```python
from build123d import *

# Parameters (mm, degrees)
F0_W     = 19.05
F0_H     = 101.6
F1_DEPTH = 9.525
F3_D     = 6.35
F5_D     = 6.35
F7_D     = 6.35


with BuildPart() as f1:
    # F0 (on Right) → F1 (new body, symmetric)
    with BuildSketch(Plane.YZ):
        Rectangle(F0_W, F0_H)
    extrude(amount=F1_DEPTH, both=True)

    # F3 (through all)
    with Locations(Plane.XZ.offset(9.525)):
        with Locations((0, 31.75), (0, -31.75)):
            Hole(F3_D / 2)

    # F5 (through all)
    with Locations(Plane.YZ.offset(9.525)):
        with Locations((0, 41.275), (0, -41.275)):
            Hole(F5_D / 2)

    # F7 (through all)
    with Locations(Plane.YZ.offset(9.525)):
        with Locations((0, -12.7)):
            Hole(F7_D / 2)


solid = f1.part
```
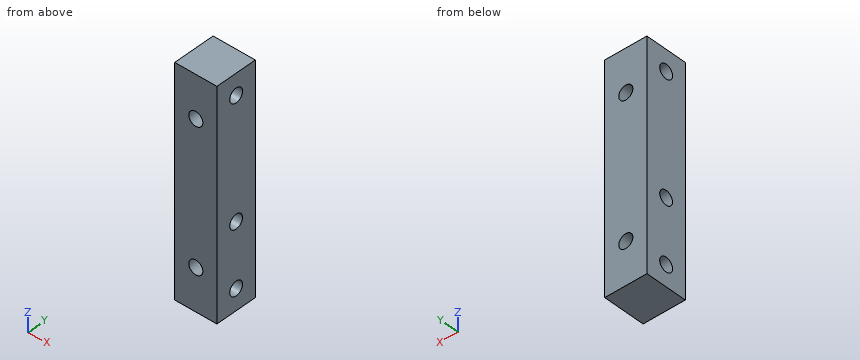
Geometry check sheet. Reference: the model listing, model coordinates, mm. Coordinates: 2 decimals unless noted, no trailing zeros. Order: outer loops, then holes, each group sorted by start corner. A loop starts at its lowest first (then second) coordinate and runs counter-clockwise, first axis right, second up.
Item 1: Scan lines: line 1 along Z through (x, y) = (-5.25, 0) (3 decimals); line 2 along Z through (x, y) = (-0.25, 0) (3 decimals); line 3 along Z through (x, y) = (-1, -4.5). Record each from-to range of solid material in increasing order.
Item 2: Depth check by flat-ended pin: pin 1 (5.5 mm diameter, centred on x = 0, z = -31.75, fed in from -Y). Enter the tip coordinate at first touch or a pass-through.
Item 3: Section check C-C (y = 5). Enter the section's corners in (x, z) (3 decimals), plus the area to 3 significant figures.
Item 4: Section check D-D (x = 7.25). Enter the section's corners in (y, z) (3 decimals).
Item 5: Section check B-B (z = -31.75). Enter the section's corners in (x, y) (3 decimals), plus the area to 3 significant figures.
Item 6: Section check A-A (y = 0). Enter the section's corners in (x, z) (3 decimals), plus the area to 3 significant figures.
Check sheet entries:
1. line 1: z = -50.8 to -44.45, -38.1 to -15.875, -9.525 to 38.1, 44.45 to 50.8
1. line 2: z = -50.8 to -44.45, -38.1 to -34.915, -28.585 to -15.875, -9.525 to 28.585, 34.915 to 38.1, 44.45 to 50.8
1. line 3: z = -50.8 to -34.76, -28.74 to 28.74, 34.76 to 50.8
2. pin 1: passes through
3. outline: (-9.525, -50.8) - (9.525, -50.8) - (9.525, 50.8) - (-9.525, 50.8) - close; hole circle Ø6.35 at (0, -31.75); hole circle Ø6.35 at (0, 31.75)
3. area: 1,870 mm2
4. outline: (-9.525, -50.8) - (9.525, -50.8) - (9.525, 50.8) - (-9.525, 50.8) - close; hole circle Ø6.35 at (0, -41.275); hole circle Ø6.35 at (0, -12.7); hole circle Ø6.35 at (0, 41.275)
5. outline: (-9.525, -9.525) - (-3.175, -9.525) - (-3.175, 9.525) - (-9.525, 9.525) - close; (3.175, -9.525) - (9.525, -9.525) - (9.525, 9.525) - (3.175, 9.525) - close
5. area: 242 mm2
6. outline: (-9.525, -50.8) - (9.525, -50.8) - (9.525, -44.45) - (-9.525, -44.45) - close; (-9.525, -38.1) - (9.525, -38.1) - (9.525, -15.875) - (-9.525, -15.875) - close; (-9.525, -9.525) - (9.525, -9.525) - (9.525, 38.1) - (-9.525, 38.1) - close; (-9.525, 44.45) - (9.525, 44.45) - (9.525, 50.8) - (-9.525, 50.8) - close; hole circle Ø6.35 at (0, -31.75); hole circle Ø6.35 at (0, 31.75)
6. area: 1,510 mm2
